Can you work these out from the drawing? Everything is in mm from the part's minimum corner. A direction names the side the tool comes from. Give positions to 0.01 mm unless a question says otherwise; leave off trailing zeros. Write each loop counter-clockwise with the first axis right and the second up, starting at its lowest first coordinate (ties: lowest second). Pieces come first, ordered by that corner, then holes. Notation, with made-up numbers: M 17,-33 L 63,-33 A27 ccw 63,-5 Z; hole C -12,41.5 d2. An arc over 180 degrees is marked long. One line per item, written item: value.
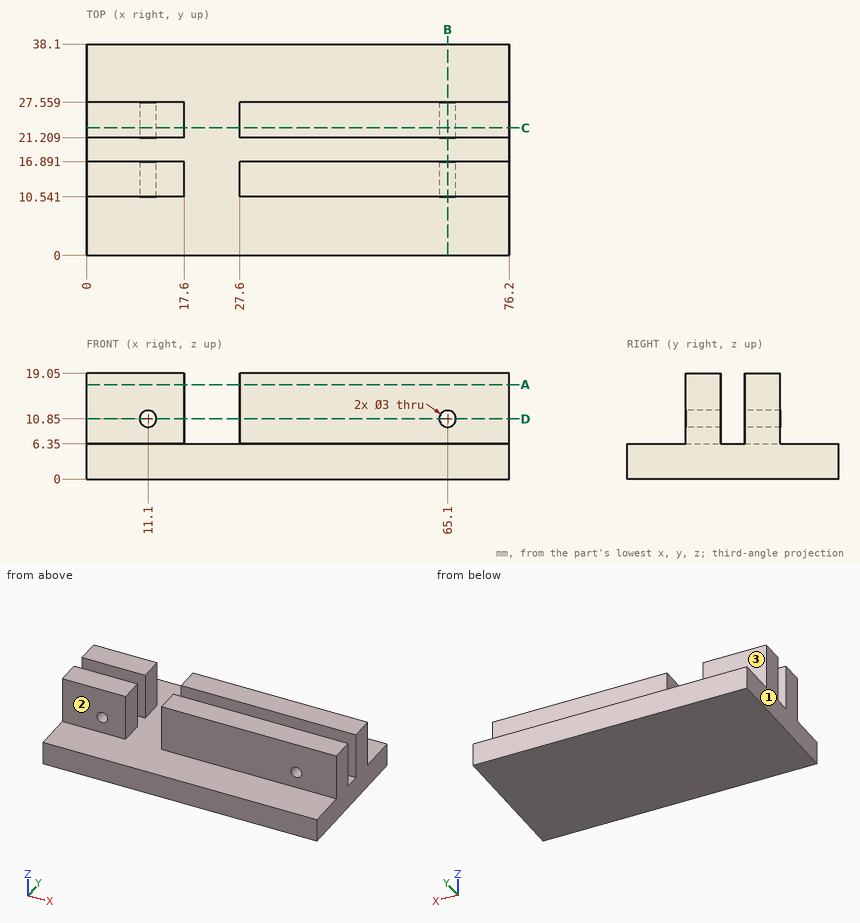
1) On a 3-axis mill with a long thin cutter (end or side, diameter ignored), from which of +Z, -Z, +X, -X, +Y, -Y can I reach the whole of each face in a straight line? I mean the marked faces 1, 2 and 3. Say none if no direction works.
Outcome:
face 1: +Z, -Z, -X, +Y, -Y
face 2: +Z, +X, -X, -Y
face 3: +Z, +X, -X, +Y
2) If we section it at A-A, the plane z = 17: Write out the boundary of the cut face in (x, y).
Outcome:
outline: M 0,10.54 L 17.6,10.54 L 17.6,16.89 L 0,16.89 Z; M 0,21.21 L 17.6,21.21 L 17.6,27.56 L 0,27.56 Z; M 27.6,10.54 L 76.2,10.54 L 76.2,16.89 L 27.6,16.89 Z; M 27.6,21.21 L 76.2,21.21 L 76.2,27.56 L 27.6,27.56 Z
3) If we section it at B-B, the plane x = 65.1: Write out the boundary of the cut face in (y, z), then the cut area to 3 significant figures.
Outcome:
outline: M 0,0 L 38.1,0 L 38.1,6.35 L 27.56,6.35 L 27.56,9.35 L 21.21,9.35 L 21.21,6.35 L 16.89,6.35 L 16.89,9.35 L 10.54,9.35 L 10.54,6.35 L 0,6.35 Z; M 10.54,12.35 L 16.89,12.35 L 16.89,19.05 L 10.54,19.05 Z; M 21.21,12.35 L 27.56,12.35 L 27.56,19.05 L 21.21,19.05 Z
area: 365 mm^2
4) I'm going to push flat-ended pins straight in: pin 1 (4 mm diameter, centred on x = 11.1, z = 10.85, fed in from -Y); pin 2 (10 mm diameter, centred on x = 12.5, z = 14.5, fed in from +Y). Where does each tip first touch, or does it pass through?
Outcome:
pin 1: stops at y = 10.54
pin 2: stops at y = 27.56
5) Please list where these lines run through material, in increasing order: L1, parallel to Y at x = 63.5, z = 15.75; L2, parallel to Z at x = 65, y = 13; L3, parallel to Z at x = 71, y = 6.5. Write a range as from..to.
Outcome:
L1: y = 10.54..16.89, 21.21..27.56
L2: z = 0..9.35, 12.35..19.05
L3: z = 0..6.35
6) If we section it at D-D, the plane z = 10.85: Give the number of separate pieces and of enclosed holes in the cut face, then the cut area to 3 significant figures.
Outcome:
separate pieces: 8
enclosed holes: 0
area: 765 mm^2
7) If we section it at C-C, the plane y = 23: Write out the boundary of the cut face in (x, z), then the cut area to 3 significant figures.
Outcome:
outline: M 0,0 L 76.2,0 L 76.2,19.05 L 27.6,19.05 L 27.6,6.35 L 17.6,6.35 L 17.6,19.05 L 0,19.05 Z; hole C 11.1,10.85 d3; hole C 65.1,10.85 d3
area: 1,310 mm^2
